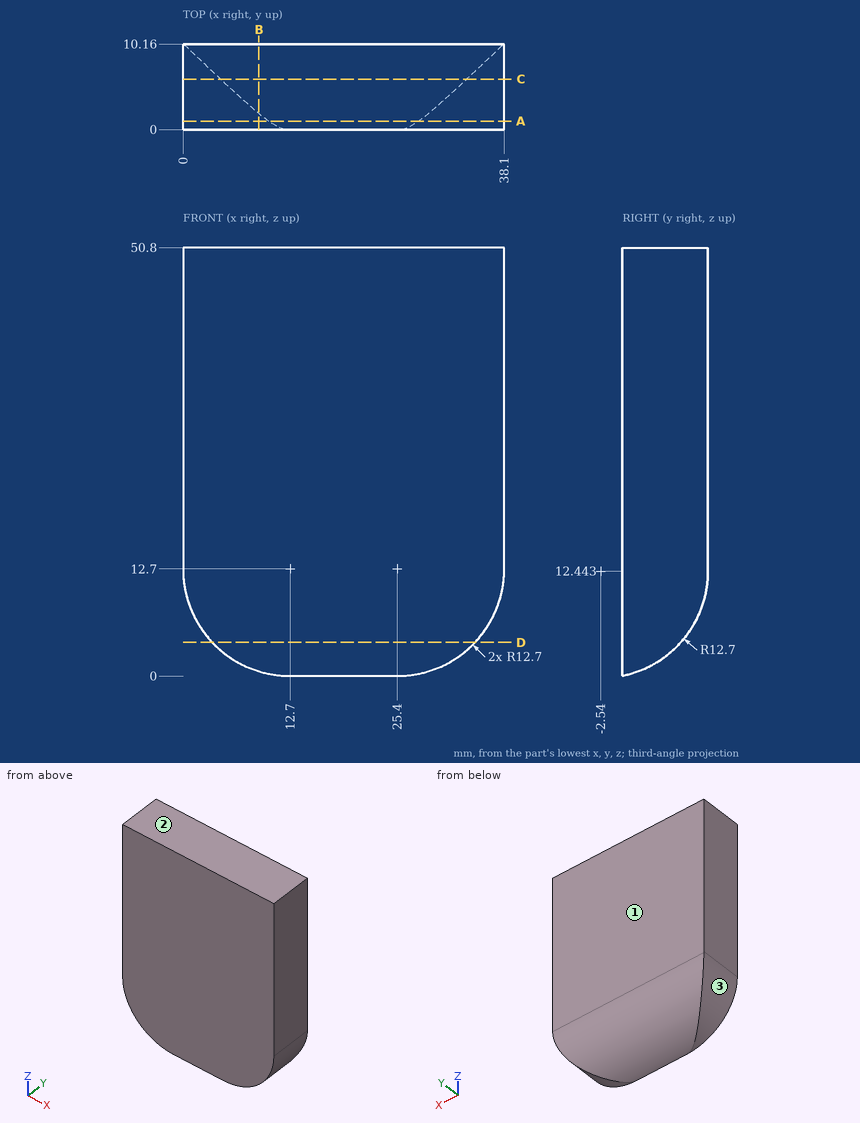
Source: three-view drawing plus pictorial views. Frame: mm from the lowest corner of the part. Give positions to 0.01 mm unless a question says otherwise; leave off trailing zeros. Write each loop counter-clockwise with the first axis right and the second up, starting at its lowest first coordinate (ties: lowest second). Pieces come first, ordered by that corner, then holes. Notation, with made-up numbers: (63, 26) - (67, 26) arc R17 cw to (67, 46) - close; hole circle Ø4 at (33.5, 41.25). An arc over 180 degrees is marked (long way). Write item = value, one per line. Start each with the question number.
Q1. Cut plane D-D, the plane z = 4. Return loops of the section in (x, y), then the cut area to 3 significant figures.
Q2. Cut plane A-A, the plane y = 1. Return loops of the section in (x, z), then the cut area to 3 significant figures.
Q3. Draft query along Z for the marked faces 1, 2 and 3. Return one class per face: +Z half, -Z half, draft (parallel to the pull), parting line (faces both ways), or undercut.
Q4. Cut plane C-C, the plane y = 6. Return loops of the section in (x, z), then the cut area to 3 significant figures.
Q5. Cut plane B-B, the plane x = 9. Return loops of the section in (y, z), then the cut area to 3 significant figures.
Q6. Material intervals for probe 1 along Z at (x, y) = (13.5, 8.75) (1 decimal); probe 2 along Y at (x, z) = (34, 11); probe 3 along Z at (x, y) = (13, 8), sorted ascending.
Computed values:
q1.outline = (3.45, 0) - (34.65, 0) - (34.65, 6.95) - (3.45, 6.95) - close
q1.area = 217 mm²
q2.outline = (0, 12.7) arc R12.7 ccw to (10.21, 0.25) - (27.89, 0.25) arc R12.7 ccw to (38.1, 12.7) - (38.1, 50.8) - (0, 50.8) - close
q2.area = 1,860 mm²
q3.face_1 = draft
q3.face_2 = +Z half
q3.face_3 = -Z half
q4.outline = (0, 12.7) arc R12.7 ccw to (4.45, 3.04) - (33.65, 3.04) arc R12.7 ccw to (38.1, 12.7) - (38.1, 50.8) - (0, 50.8) - close
q4.area = 1,790 mm²
q5.outline = (0, 0.55) - (1.92, 0.55) arc R12.7 ccw to (10.16, 12.44) - (10.16, 50.8) - (0, 50.8) - close
q5.area = 484 mm²
q6.probe_1 = 6.6 to 50.8
q6.probe_2 = 0 to 10.08
q6.probe_3 = 5.36 to 50.8
